Here's how the part is built. I have some questions about the finished solid (model axes, mm). A direction names the side the tool comes from. Coordinates: 2 decimals unless noted, no trailing zeros. Order: outer loops, then holes, each group sorted by start corner. A loop starts at its lowest first (then second) coordinate and runs counter-clockwise, first axis right, second up. Notation, with made-up numbers: M 56,41 L 101,41 A17 ccw 101,53 Z; hole C 22.25,30.25 d5. An arc over 180 degrees is marked long. One line per question, with ' | ' between items. Start each with the question number.
Autodesk Inventor part; units mm, degrees
ref_plane "YZ Plane" through (0, 0, 0) normal (1, 0, 0) x (0, 1, 0)
ref_plane "XZ Plane" through (0, 0, 0) normal (0, 1, 0) x (-1, 0, 0)
ref_plane "XY Plane" through (0, 0, 0) normal (0, 0, 1) x (1, 0, 0)
sketch "Sketch1" plane through (0, 0, 0) normal (1, 0, 0) x (0, 1, 0)
  line L0 (0, 0) -> (70, 0)
  line L1 (70, 0) -> (70, -34)
  line L2 (70, -34) -> (0, -34)
  line L3 (0, -34) -> (0, 0)
  dimension "d0" = 34
  dimension "d1" = 70
extrude "Extrusion1" add sketch "Sketch1" along normal blind 2.5
fillet "Fillet1" radius 2 2 edges at (1.25, 70, -34) (1.25, 0, -34)
fillet "Fillet2" radius 0.5 10 edges at (2.5, 69.4142, -33.4142) (2.5, 70, -16) (2.5, 0.5858, -33.4142) (2.5, 0, -16) (2.5, 35, -34) (0, 0.5858, -33.4142) (0, 35, -34) (0, 69.4142, -33.4142) (0, 70, -16) (0, 0, -16)
sketch "Sketch2" plane through (0, 0, 0) normal (-1, 0, 0) x (0, 0, 1)
  line L0 (0, 69.5) -> (0, 0.5)
  line L1 (7, 40) -> (-7, 40)
  line L2 (-7, 40) -> (-7, 30)
  line L3 (-7, 30) -> (7, 30)
  line L4 (7, 30) -> (7, 40)
  line L5 (0, 69.5) -> (0, 0.5)
  line L6 (7, 40) -> (-7, 30) construction
  line L7 (-7, 40) -> (7, 30) construction
  line L8 (-3, 40) -> (-3, 30)
  point P0 (0, 0)
  point P1 (0, 35)
  point P2 (-7, 35)
  point P3 (-3, 35)
  dimension "d6" = 10
  dimension "d7" = 14
  dimension "d8" = 4
extrude "Extrusion2" add sketch "Sketch2" along normal blind 5 contours L8 L3 L2 L1
fillet "Fillet3" radius 2 4 edges at (-2.5, 40, -3) (-2.5, 30, -3) (-2.5, 30, -7) (-2.5, 40, -7)
fillet "Fillet4" radius 0.5 4 edges at (-5, 30.5856, -3.5856) (-5, 35, -3) (-5, 39.4144, -3.5856) (-5, 35, -7)
sketch "Sketch3" plane through (0, 0.5, 0) normal (0, 0, 1) x (1, 0, 0)
  arc A0 (2.5, 69) -> (2, 69.5) centre (2, 69) ccw
  arc A1 (0.5, 69.5) -> (0, 69) centre (0.5, 69) ccw
  arc A2 (0.5, 69.5) -> (0, 69) centre (0.5, 69) ccw
  line L0 (0, 69) -> (0, 0)
  arc A3 (0, 0) -> (0.5, -0.5) centre (0.5, 0) ccw
  line L1 (0.5, -0.5) -> (2, -0.5)
  arc A4 (2, -0.5) -> (2.5, 0) centre (2, 0) ccw
  line L2 (2.5, 69) -> (2.5, 0)
  arc A5 (2.5, 69) -> (2, 69.5) centre (2, 69) ccw
  line L3 (0.5, 69.5) -> (2, 69.5)
  point P0 (0, -0.5)
  point P1 (0, 69)
extrude "Extrusion3" add sketch "Sketch3" along normal blind 20
properties part number "tapa de caja de servomotores"
1. Imagine slicing it at A-A (y = 33.5). List the corners of the cut face in (x, z) for me, then the cut area to 3 significant figures.
2. Which directions (+Z, -Z, +X, -X, +Y, -Y) give clear straight access to the entire face, cutting with the end or side of a thin tool? Please do faces 1 (the face through (-2.28, 30.6, -6.43)), 2 (the face through (-2, 35, -3)), 3 (the face through (-2.28, 30.57, -3.6)), 4 (the face through (-2, 35, -7)).
3. I need wall thicknesses on line 1 (X direction, y = 56, z = 16); line 2 (Y direction, x = -1.25, z = -6.5); line 3 (Z direction, x = 0.25, y = 23.5). Which ranges of each line are inside material? Lowest first, please.
4. Imagine slicing it at D-D (y = 25). List the corners of the cut face in (x, z) for me, then the cut area to 3 significant figures.
5. Imagine slicing it at C-C (z = 4). List the corners of the cut face in (x, y) for me, then the cut area to 3 significant figures.
6. Will these pins go through, and if not, where does the flat tip stop? pin 1 (1 mm diameter, centred on y = 20, z = -22.5, fed in from -X); pin 2 (2 mm diameter, centred on x = -3, y = 35, fed in from -Z).
Entries:
1) outline: M -5,-6.5 A0.5 ccw -4.5,-7 L 0,-7 L 0,-33.5 A0.5 ccw 0.5,-34 L 2,-34 A0.5 ccw 2.5,-33.5 L 2.5,20 L 0,20 L 0,-3 L -4.5,-3 A0.5 ccw -5,-3.5 Z | area: 155 mm²
2) face 1: -Z, -X, -Y | face 2: +Z, -X, +Y, -Y | face 3: +Z, -X, -Y | face 4: -Z, -X, +Y, -Y
3) line 1: 0 to 2.5 | line 2: 30.68 to 39.32 | line 3: -33.93 to 20
4) outline: M 0,-33.5 A0.5 ccw 0.5,-34 L 2,-34 A0.5 ccw 2.5,-33.5 L 2.5,20 L 0,20 Z | area: 135 mm²
5) outline: M 0,0.5 A0.5 ccw 0.5,0 L 2,0 A0.5 ccw 2.5,0.5 L 2.5,69.5 A0.5 ccw 2,70 L 0.5,70 A0.5 ccw 0,69.5 Z | area: 175 mm²
6) pin 1: x = 0 | pin 2: z = -7
